CAD build for the part. Positions are in the model's coordinates, mm. A direction names the side the tool comes from. Give positions to 0.01 mm unless a question says otherwise; leave off trailing zeros. Loops run counter-clockwise (first coordinate to the right, second up) from the corner with the lowest first, then second, coordinate; pieces in that order, holes last. Notation, with made-up numbers: (-16.75, 28.5) - (34.25, 28.5) arc R17 cw to (34.25, 42.5) - close; hole circle Ø7 at (31.25, 29). An arc over 180 degrees is marked (long way). Return JSON: item names as keys, results as strings.
from build123d import *

# Parameters (mm, degrees)
F0_W     = 390.525
F0_H     = 158.75
F1_DEPTH = 19.05
F3_DEPTH = 558.8
F4_W     = 307.975
F4_H     = 533.4
F5_DEPTH = 88.9


with BuildPart() as f1:
    # F0 (on Front) → F1 (new body)
    with BuildSketch(Plane.XZ):
        Rectangle(F0_W, F0_H)
    extrude(amount=F1_DEPTH)

    # F2 (on face) → F3 (join)
    with BuildSketch(Plane(origin=(0, 0, 0), x_dir=(-1, 0, 0), z_dir=(0, 1, 0))):
        Polygon((-166.6875, -66.675), (0, -66.675), (166.6875, -66.675), (166.6875, 34.925), (-166.6875, 34.925), align=None)
    extrude(amount=F3_DEPTH)

    # F4 (on face) → F5 (cut)
    with BuildSketch(Plane.XY.offset(34.925)):
        with Locations((0, 279.4)):
            Rectangle(F4_W, F4_H)
    extrude(amount=-F5_DEPTH, mode=Mode.SUBTRACT)


solid = f1.part
1. Cut at C-C, the plane y = 272.5. Write the cut outline in (x, z) (1 decimal), plus the area to 3 significant figures.
Values follow:
{"outline": "(-166.7, -66.7) - (166.7, -66.7) - (166.7, 34.9) - (154, 34.9) - (154, -54) - (-154, -54) - (-154, 34.9) - (-166.7, 34.9) - close", "area": "6,490 mm²"}
2. Pull direction Y, two halves, no side cores. Call faces 6 (the face through (-3, -19.05, 1)), 7 (the face through (-2, 12.7, -9)), 8 (the face through (2, 558.8, -15)), 9 (the face through (2, 275, -66.675)): +Y half, -Y half, draft (parallel to the pull), parting line (faces both ways), or undercut.
Values follow:
{"face 6": "-Y half", "face 7": "undercut", "face 8": "+Y half", "face 9": "draft"}
3. Cut at B-B, the plane x = 56. Write the cut outline in (y, z) (3 decimals), plus the area to 3 significant figures.
Values follow:
{"outline": "(-19.05, -79.375) - (0, -79.375) - (0, -66.675) - (558.8, -66.675) - (558.8, 34.925) - (546.1, 34.925) - (546.1, -53.975) - (12.7, -53.975) - (12.7, 34.925) - (0, 34.925) - (0, 79.375) - (-19.05, 79.375) - close", "area": "12,400 mm²"}
4. Which spindle directions (+Z, -Z, +X, -X, +Y, -Y) get a long thin tool onto all of the face, cutting with end or side? Do faces 1 (the face through (153.988, 276, -9)), 2 (the face through (166.688, 275, -15)), 3 (the face through (-166.688, 275, -17)), 4 (the face through (-161, 278, 34.925)), 5 (the face through (-195.262, -9, -1)). Say none if no direction does.
Values follow:
{"face 1": "+Z", "face 2": "+Z, -Z, +X, +Y", "face 3": "+Z, -Z, -X, +Y", "face 4": "+Z, +X, -X, +Y", "face 5": "+Z, -Z, -X, +Y, -Y"}
5. Cut at D-D, the plane z = 62.5. Write the cut outline in (x, y).
Values follow:
{"outline": "(-195.26, -19.05) - (195.26, -19.05) - (195.26, 0) - (-195.26, 0) - close"}
6. Drop flat-ended pins along their axis: P1, Ø12, axis at x = 95, y = 464.5, coming from the +Z side (3 decimals); P2, Ø8, axis at y = 161.5, z = -59, coming from the -X side; P3, Ø10, axis at x = -129.5, y = 280.5, coming from the -Z side (3 decimals). Give the stop position or say it passes through.
Values follow:
{"P1": "stops at z = -53.975", "P2": "stops at x = -166.69", "P3": "stops at z = -66.675"}
7. Drill centre lines: probe 1 along Y at (x, z) = (-29, -35.5); probe 2 along X at (y, z) = (55, 7.5); probe 3 along Z at (x, y) = (126, 155.5) (3 decimals). Where is each one in solid material? Low to high.
Values follow:
{"probe 1": "y = -19.05 to 12.7, 546.1 to 558.8", "probe 2": "x = -166.69 to -153.99, 153.99 to 166.69", "probe 3": "z = -66.675 to -53.975"}
8. Cut at A-A, the plane z = -35.5. Write the cut outline in (x, y), plus the area to 3 significant figures.
Values follow:
{"outline": "(-195.26, -19.05) - (195.26, -19.05) - (195.26, 0) - (166.69, 0) - (166.69, 558.8) - (-166.69, 558.8) - (-166.69, 0) - (-195.26, 0) - close; hole (-153.99, 12.7) - (153.99, 12.7) - (153.99, 546.1) - (-153.99, 546.1) - close", "area": "29,500 mm²"}
